```python
from build123d import *

# Parameters (mm, degrees)
F1_DEPTH = 10.16


with BuildPart() as f1:
    # F0 (on Top) → F1 (new body)
    with BuildSketch(Plane.XY):
        Polygon((31.75, 0), (19.05, 0), (19.05, -10.16), (0, -10.16), (0, -25.4), (10.16, -25.4), (10.16, -38.1), (0, -38.1), (0, -50.8), (10.16, -50.8), (10.16, -63.5), (0, -63.5), (0, -76.2), (10.16, -76.2), (10.16, -88.9), (0, -88.9), (0, -104.14), (19.05, -104.14), (19.05, -114.3), (31.75, -114.3), (31.75, -104.14), (44.45, -104.14), (44.45, -114.3), (57.15, -114.3), (57.15, -104.14), (69.85, -104.14), (69.85, -114.3), (82.55, -114.3), (82.55, -104.14), (95.25, -104.14), (95.25, -114.3), (107.95, -114.3), (107.95, -104.14), (120.65, -104.14), (120.65, -114.3), (133.35, -114.3), (133.35, -104.14), (146.05, -104.14), (146.05, -114.3), (158.75, -114.3), (158.75, -104.14), (171.45, -104.14), (171.45, -114.3), (184.15, -114.3), (184.15, -104.14), (203.2, -104.14), (203.2, -88.9), (193.04, -88.9), (193.04, -76.2), (203.2, -76.2), (203.2, -63.5), (193.04, -63.5), (193.04, -50.8), (203.2, -50.8), (203.2, -38.1), (193.04, -38.1), (193.04, -25.4), (203.2, -25.4), (203.2, -10.16), (184.15, -10.16), (184.15, 0), (171.45, 0), (171.45, -10.16), (158.75, -10.16), (158.75, 0), (146.05, 0), (146.05, -10.16), (133.35, -10.16), (133.35, 0), (120.65, 0), (120.65, -10.16), (107.95, -10.16), (107.95, 0), (95.25, 0), (95.25, -10.16), (82.55, -10.16), (82.55, 0), (69.85, 0), (69.85, -10.16), (57.15, -10.16), (57.15, 0), (44.45, 0), (44.45, -10.16), (31.75, -10.16), align=None)
    extrude(amount=F1_DEPTH)


solid = f1.part
```
For this review, take the finished solid that the model builds, in its own axes (mm). A direction names the side the tool comes from. Give positions to 0.01 mm unless a question says otherwise; leave off trailing zeros. Write each loop counter-clockwise with the first axis right and the second up, starting at its lowest first coordinate (ties: lowest second). Pieces come first, ordered by that corner, then holes. Notation, with made-up numbers: M -38.5,85 L 1.5,85 A9 cw 1.5,95 Z; hole C 78,-14 d11. An arc over 180 degrees is marked long. Answer as CSV lines item,"result".
1. Draft analysis for pull direction Y (two halves, no side actions). For faces 4 (the flat face through (89, -10.16, 5)), 5 (the flat face through (193.04, -83, 5)), 6 (the flat face through (95.25, -5, 5)), 7 (the flat face through (25, -114.3, 5)), state which applies: +Y half, -Y half, draft (parallel to the pull), parting line (faces both ways), or undercut.
Findings:
face 4,"+Y half"
face 5,"undercut"
face 6,"draft"
face 7,"-Y half"
2. Consider section A-A, the plane y = -81. Write out the cut boundary in (x, z), then the cut area to 3 significant figures.
Findings:
outline,"M 10.16,0 L 193.04,0 L 193.04,10.16 L 10.16,10.16 Z"
area,"1,860 mm2"
3. Consider section B-B, the plane x = 92. Write out the cut boundary in (y, z).
Findings:
outline,"M -104.14,0 L -10.16,0 L -10.16,10.16 L -104.14,10.16 Z"
4. For pin 1 (5 mm diameter, centred on y = -54, z = 7, fed in from +X); pin 2 (5 mm diameter, centred on y = -108, z = 3, fed in from -X); pin 3 (5 mm diameter, centred on x = 196, z = 4.5, fed in from -Y), all flat-tipped, find the tip position at first contact; note any pin that passes through.
Findings:
pin 1,"stops at x = 193.04"
pin 2,"stops at x = 19.05"
pin 3,"stops at y = -104.14"
5. For faces 1 (the flat face through (82.55, -109, 5)), 2 (the flat face through (193.04, -57, 5)), 3 (the flat face through (133.35, -5, 5)), list the 3-axis set-ups (+Z, -Z, +X, -X, +Y, -Y) from which the entire face can be reached by the end or side of a thin tool; tool diameter is ignored.
Findings:
face 1,"+Z, -Z, -Y"
face 2,"+Z, -Z, +X"
face 3,"+Z, -Z, +Y"
6. Wall thickness on line 1 (Y direction, x = 167, z = 2.25); line 2 (X direction, y = -34, z = 2): over which ranges is each line inside the solid? List them lowest first.
Findings:
line 1,"y = -104.14 to -10.16"
line 2,"x = 10.16 to 193.04"
